Source: three-view drawing plus pictorial views. Frame: mm from the lowest corner of the part. A direction names the side the tool comes from. Give positions to 0.01 mm unless a question says otherwise; leave off trailing zeros. Write each loop counter-clockwise with the first axis right and the second up, starting at its lowest first coordinate (ties: lowest second). Pieces come first, ordered by that corner, then holes. Notation, with made-up numbers: (7, -0.75) -> (64, -0.75) arc R22 ccw to (64, 35.25) -> close; hole circle Ø9 at (14.5, 13). An arc over 180 degrees is marked (long way). Answer in a Markdown table with one row per item. Add a question column.
Item 1: First-contact query: P1, Ø2, axis at x = 10, y = 3.15, coming from the -Z side; P2, Ø0.9, axis at y = 2.5, z = 3.5, coming from the -X side; P3, Ø2.5, axis at y = 3, z = 3, coming from the +X side; P4, Ø3, axis at x = 17, y = 2, coming from the -Z side. Flat tips, straight axial feed; report the tip coordinate or a pass-through.
Item 2: Section query C-C on y = 3.15. State how many separate pieces and enclosed holes the cut face has, plus the area to 3 significant figures.
Item 3: Material intervals for probe 1 along Y at (x, z) = (17.7, 19) (3 decimals); probe 2 along X at (y, z) = (3.15, 8.5); probe 3 along Z at (x, y) = (8.25, 3.75), sorted ascending. Write a range as from..to.
Item 4: Access query for the marked faces 4, 5 and 6. Directions: +Z, -Z, +X, -X, +Y, -Y. A direction counts if a zero-diameter tool reaches every point of the face in a straight line with its end or side. Return the directions, or none.
Item 5: Draft query along X for the marked faces 1, 2 and 3. Return one class per face: +X half, -X half, draft (parallel to the pull), parting line (faces both ways), or undercut.
Item 6: Section query D-D on x = 10. Output: boundary loops of the cut face in (y, z).
Item 7: Section query A-A on x = 8. Output: boundary loops of the cut face in (y, z), plus the area to 3 significant figures.
Item 8: Section query B-B on z = 17. Output: boundary loops of the cut face in (x, y).
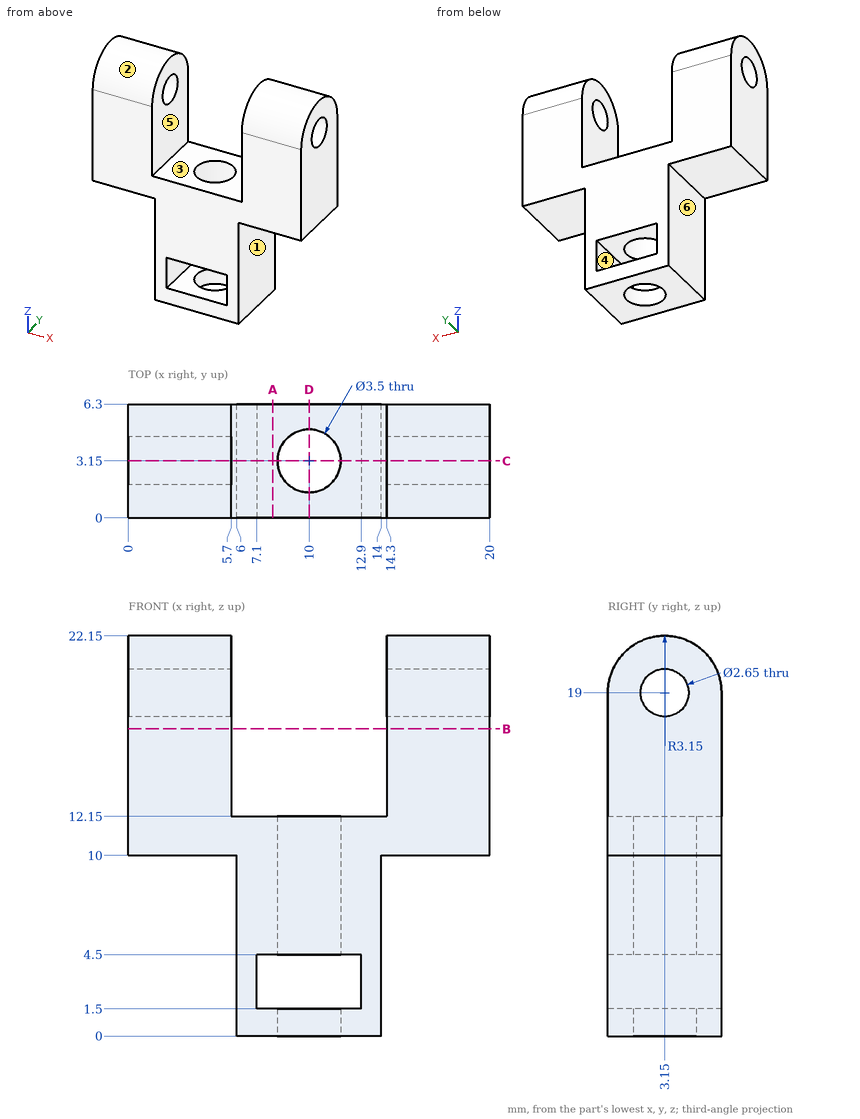
Findings below:
| question | item | result |
|---|---|---|
| 1 | P1 | passes through |
| 1 | P2 | stops at x = 6 |
| 1 | P3 | stops at x = 14 |
| 1 | P4 | stops at z = 10 |
| 2 | separate pieces | 4 |
| 2 | enclosed holes | 0 |
| 2 | area | 157 mm^2 |
| 3 | probe 1 | y = 0..1.825, 4.475..6.3 |
| 3 | probe 2 | x = 6..8.25, 11.75..14 |
| 3 | probe 3 | z = 0..1.5, 4.5..12.15 |
| 4 | face 4 | +Y, -Y |
| 4 | face 5 | +Z, +Y, -Y |
| 4 | face 6 | -Z, -X, +Y, -Y |
| 5 | face 1 | +X half |
| 5 | face 2 | draft |
| 5 | face 3 | undercut |
| 6 | outline | (0, 0) -> (1.4, 0) -> (1.4, 1.5) -> (0, 1.5) -> close; (0, 4.5) -> (1.4, 4.5) -> (1.4, 12.15) -> (0, 12.15) -> close; (4.9, 0) -> (6.3, 0) -> (6.3, 1.5) -> (4.9, 1.5) -> close; (4.9, 4.5) -> (6.3, 4.5) -> (6.3, 12.15) -> (4.9, 12.15) -> close |
| 7 | outline | (0, 0) -> (6.3, 0) -> (6.3, 1.5) -> (0, 1.5) -> close; (0, 4.5) -> (6.3, 4.5) -> (6.3, 12.15) -> (0, 12.15) -> close |
| 7 | area | 57.6 mm^2 |
| 8 | outline | (0, 0) -> (5.7, 0) -> (5.7, 6.3) -> (0, 6.3) -> close; (14.3, 0) -> (20, 0) -> (20, 6.3) -> (14.3, 6.3) -> close |
